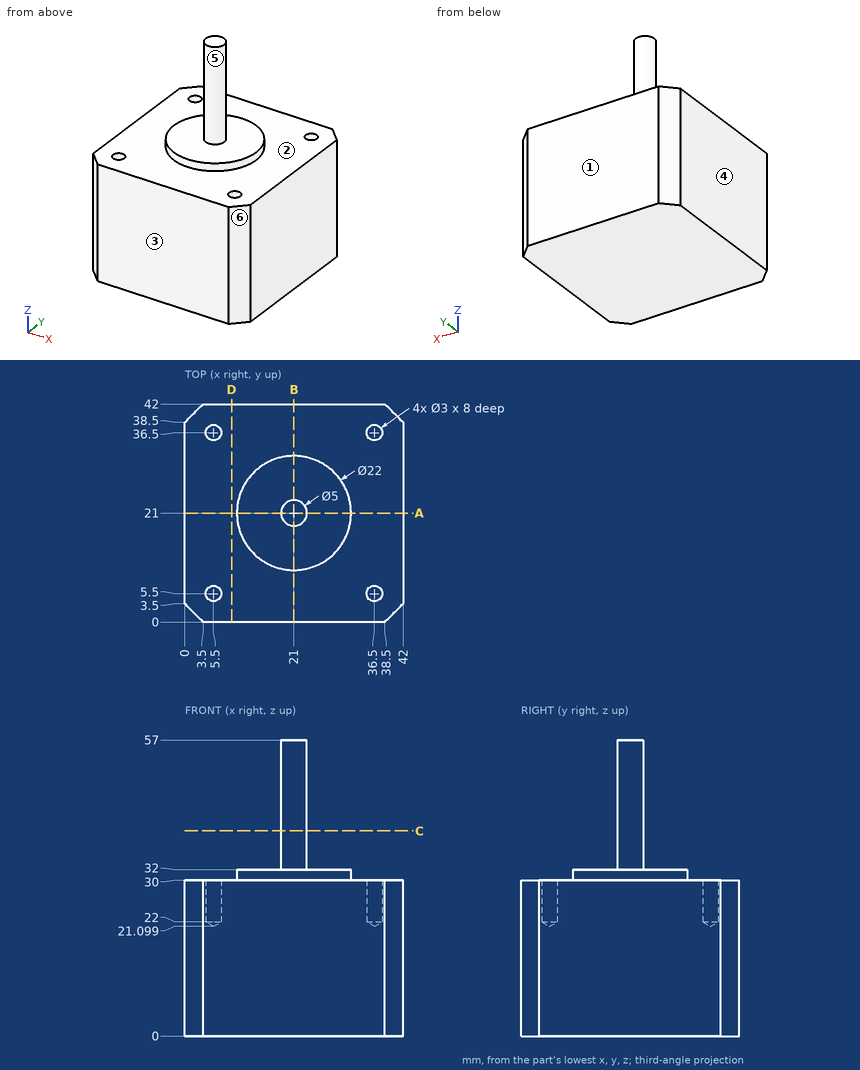
Geometry check sheet. Reference: drawing and pictorial views, mm from the part's lowest x, y, z. A direction names the side the tool comes from. Coordinates: 2 decimals unless noted, no trailing zeros. Write each loop counter-clockwise with the first axis right and the second up, starting at its lowest first coordinate (ties: lowest second). Pieces come first, ordered by that corner, then holes. Notation, with made-up numbers: M 42,-9.75 L 98,-9.75 A23 ccw 98,13.25 Z; hole C 47.5,-23.5 d2. An arc over 180 degrees is marked long. Use one line per item in the form item = value.
Item 1: Set-up check for the marked faces 1 and 2: record each of +Z, -Z, +X, -X, +Y, -Y from which the full face is reachable in a straight line by a thin tool's end or side.
Answer below:
face_1 = +Z, -Z, +X, -X, +Y
face_2 = +Z
Item 2: Sectioned sample at D-D, the plane x = 9. Record the cut outline in (y, z), and give its area (3 significant figures).
Answer below:
outline = M 0,0 L 42,0 L 42,30 L 0,30 Z
area = 1,260 mm^2
Item 3: Sectioned sample at C-C, the plane z = 39.5. Record the cut outline in (x, y).
Answer below:
outline = C 21,21 d5
Item 4: Sectioned sample at A-A, the plane y = 21. Record the cut outline in (x, z), and give its area (3 significant figures).
Answer below:
outline = M 0,0 L 42,0 L 42,30 L 32,30 L 32,32 L 23.5,32 L 23.5,57 L 18.5,57 L 18.5,32 L 10,32 L 10,30 L 0,30 Z
area = 1,430 mm^2
Item 5: Gauge pin test, flat ends, axial feed: pin 1 Ø2 at (x, y) = (25, 10.5) entering from +Z; pin 2 Ø12 at (x, y) = (6.5, 31.5) entering from -Z; pin 3 Ø3.5 at (x, y) = (36.5, 5.5) entering from +Z; pin 4 Ø2.5 at (x, y) = (5.5, 36.5) entering from +Z. Record the tip position at first contact, or that the pin passes through.
Answer below:
pin_1 = 32
pin_2 = 0
pin_3 = 30
pin_4 = 21.85
Item 6: Material ranges on L1, parallel to Y at x = 5.5, z = 24; L2, parallel to Y at x = 36, z = 24 (1 decimal), recorded low to high. Write a range as from..to.
Answer below:
L1 = 0..4, 7..35, 38..42
L2 = 0..4.1, 6.9..35.1, 37.9..42
Item 7: Release check for a two-part mould opening along X. For the marked faces 3, 4, 5 and 6 record: pulls with the +X half, pulls with the -X half, needs draft (parallel to the pull), parting line crosses it, or undercut.
Answer below:
face_3 = needs draft
face_4 = pulls with the -X half
face_5 = parting line crosses it
face_6 = pulls with the +X half
